```python
from build123d import *

# Parameters (mm, degrees)
BOSS_EXTRUDE1_DEPTH = 45
SKETCH2_R           = 1.5
CUT_EXTRUDE1_DEPTH  = 5
CUT_EXTRUDE3_DEPTH  = 45


with BuildPart() as part:
    # Sketch1 → Boss-Extrude1 (new body)
    with BuildSketch(Plane(origin=(0, 0, 0), x_dir=(1, 0, 0), z_dir=(0, 1, 0))):
        Polygon((-21.15, 14.15), (-14.15, 21.15), (14.15, 21.15), (21.15, 14.15), (21.15, -14.15), (14.15, -21.15), (-14.15, -21.15), (-21.15, -14.15), align=None)
    extrude(amount=BOSS_EXTRUDE1_DEPTH)

    # Sketch2 → Cut-Extrude1 (cut)
    with BuildSketch(Plane(origin=(0, 45, 0), x_dir=(1, 0, 0), z_dir=(0, 1, 0))):
        with Locations((-15.5, 15.5)):
            Circle(SKETCH2_R)
        with Locations((15.5, 15.5)):
            Circle(SKETCH2_R)
        with Locations((-15.5, -15.5)):
            Circle(SKETCH2_R)
        with Locations((15.5, -15.5)):
            Circle(SKETCH2_R)
    extrude(amount=-CUT_EXTRUDE1_DEPTH, mode=Mode.SUBTRACT)

    # Sketch3 → Cut-Extrude3 (cut)
    with BuildSketch(Plane(origin=(0, 45, 0), x_dir=(1, 0, 0), z_dir=(0, 1, 0))):
        Polygon((-15, 11), (-11, 15), (11, 15), (15, 11), (15, -11), (11, -15), (-11, -15), (-15, -11), align=None)
    extrude(amount=-CUT_EXTRUDE3_DEPTH, mode=Mode.SUBTRACT)


solid = part.part
```
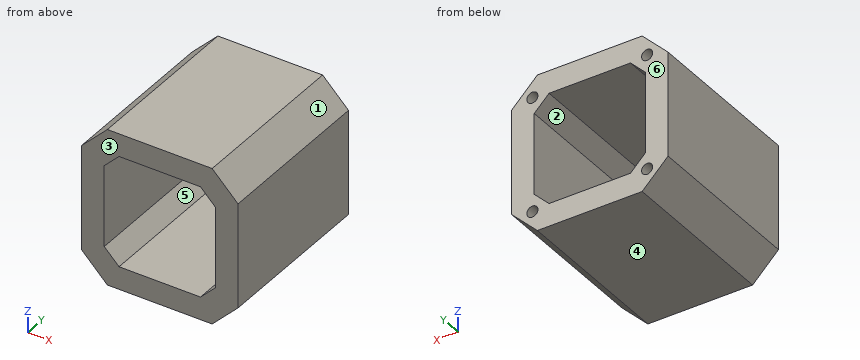
Read the model definition and answer for the solid it produces. Units are mm, in the model's axes. Face numbers are marked on the shaded views. A direction names the side the tool comes from. Round coordinates to 2 decimals unless told otherwise and drop trailing zeros. Write each loop counter-clockwise with the first axis right and the second up, starting at its lowest first coordinate (ties: lowest second). Pieces come first, ordered by that corner, then holes. Notation, with made-up numbers: (-34, 88.5) - (11, 88.5) arc R15 ccw to (11, 114.5) - close; hole circle Ø8 at (83.5, -19.5). An arc over 180 degrees is marked (long way). One line per item, written item: value.
Q1. Find section B-B (y = 33). Determine the outline of the cut face in (x, z).
The answers:
outline: (-21.15, -14.15) - (-14.15, -21.15) - (14.15, -21.15) - (21.15, -14.15) - (21.15, 14.15) - (14.15, 21.15) - (-14.15, 21.15) - (-21.15, 14.15) - close; hole (-15, -11) - (-11, -15) - (11, -15) - (15, -11) - (15, 11) - (11, 15) - (-11, 15) - (-15, 11) - close
Q2. This flat-tipped pin is pushed along its axis until it touches: P1, Ø0.9, axis at x = 15, z = -15, coming from the +Y side. Where does it stop, or does it pass through?
The answers:
P1: stops at y = 40
Q3. Find section C-C (x = -9.5). Determine the outline of the cut face in (y, z).
The answers:
outline: (0, -21.15) - (45, -21.15) - (45, -15) - (0, -15) - close; (0, 15) - (45, 15) - (45, 21.15) - (0, 21.15) - close
Q4. Find section D-D (x = -18). Determine the outline of the cut face in (y, z), and give its area (3 significant figures).
The answers:
outline: (0, -17.3) - (45, -17.3) - (45, 17.3) - (0, 17.3) - close
area: 1,560 mm2
Q5. For a pull along Z with two mould halves and no side action, classify the marked faces 1, 2, 3 and 4 as pulls with the +Z half, pulls with the -Z half, needs draft (parallel to the pull), parting line crosses it, or undercut.
The answers:
face 1: pulls with the +Z half
face 2: undercut
face 3: needs draft
face 4: pulls with the -Z half
Q6. Which of the six approach directions +Z, -Z, +X, -X, +Y, -Y give full straight-line access (tool end or side, diameter ignored) to the marked faces 5 and 6?
The answers:
face 5: +Y, -Y
face 6: +Z, -Z, +X, -X, +Y
Q7. Straight lines are drawn through the part: line 1 (Z direction, x = -6, y = 10); line 2 (X direction, y = 41.5, z = 16); line 3 (X direction, y = 43, z = 15.5). For each, find the intervals that lie inside material, in ascending order. Write a range as from..to.
The answers:
line 1: z = -21.15..-15, 15..21.15
line 2: x = -19.3..-16.91, -14.09..14.09, 16.91..19.3
line 3: x = -19.8..-17, -14..14, 17..19.8
Q8. Find section A-A (z = -5.5). Determine the outline of the cut face in (x, y), and give its area (4 significant figures).
The answers:
outline: (-21.15, 0) - (-15, 0) - (-15, 45) - (-21.15, 45) - close; (15, 0) - (21.15, 0) - (21.15, 45) - (15, 45) - close
area: 553.5 mm2
